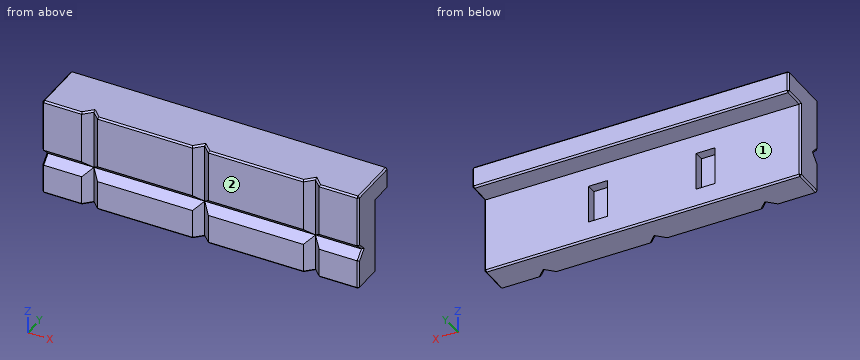
```python
from build123d import *

# Parameters (mm, degrees)
PAD_DEPTH         = 50
POCKET_DEPTH      = 24.001
POCKET_DEPTH_BACK = -7.001
SKETCH002_W       = 6
SKETCH002_H       = 12
POCKET001_DEPTH   = 3
CHAMFER_SIZE      = 0.5


with BuildPart() as part:
    # Sketch → Pad (new body, symmetric)
    with BuildSketch(Plane.YZ):
        Polygon((7, 7), (-10, 7), (-10, -9.5), (-7.5, -12), (-10, -14.5), (-10, -24), (0, -24), (0, 0), (7, 0), align=None)
    extrude(amount=PAD_DEPTH, both=True)

    # Sketch001 → Pocket (cut, two sides)
    with BuildSketch(Plane.XY) as pocket_sk:
        Polygon((-37.5, -10), (-32.5, -10), (-35, -7.5), align=None)
        Polygon((-2.5, -10), (2.5, -10), (0, -7.5), align=None)
        Polygon((32.5, -10), (37.5, -10), (35, -7.5), align=None)
    extrude(amount=-POCKET_DEPTH, mode=Mode.SUBTRACT)
    extrude(pocket_sk.sketch, amount=-POCKET_DEPTH_BACK, mode=Mode.SUBTRACT)

    # Sketch002 → Pocket001 (cut)
    with BuildSketch(Plane.XZ):
        with Locations((-20, -12)):
            Rectangle(SKETCH002_W, SKETCH002_H)
        with Locations((14, -12)):
            Rectangle(SKETCH002_W, SKETCH002_H)
    extrude(amount=POCKET001_DEPTH, mode=Mode.SUBTRACT)

    # Chamfer
    chamfer_edges = [part.edges().sort_by_distance(p)[0] for p in [
        (50, -1.5, 7),
        (50, -10, -1.25),
        (50, -8.75, -10.75),
        (50, -8.75, -13.25),
        (50, -10, -19.25),
        (50, -5, -24),
        (50, 0, -12),
        (50, 3.5, 0),
        (50, 7, 3.5),
        (-50, -1.5, 7),
        (-50, -10, -1.25),
        (-50, -8.75, -10.75),
        (-50, -8.75, -13.25),
        (-50, -10, -19.25),
        (-50, -5, -24),
        (-50, 0, -12),
        (-50, 3.5, 0),
        (-50, 7, 3.5),
        (0, 7, 0),
        (0, 7, 7),
        (-43.75, -10, 7),
        (-36.25, -8.75, 7),
        (-33.75, -8.75, 7),
        (-17.5, -10, 7),
        (-1.25, -8.75, 7),
        (1.25, -8.75, 7),
        (17.5, -10, 7),
        (33.75, -8.75, 7),
        (36.25, -8.75, 7),
        (43.75, -10, 7),
        (0, 0, -24),
        (43.75, -10, -24),
        (36.25, -8.75, -24),
        (33.75, -8.75, -24),
        (17.5, -10, -24),
        (1.25, -8.75, -24),
        (-1.25, -8.75, -24),
        (-17.5, -10, -24),
        (-33.75, -8.75, -24),
        (-36.25, -8.75, -24),
        (-43.75, -10, -24),
    ]]
    chamfer(chamfer_edges, length=CHAMFER_SIZE)


solid = part.part
```
Check sheet for the modelled part. Datum: model origin and axes. Units: mm. Face numbers are marked on the shaded views. A direction names the side the tool comes from. Coordinates: 2 decimals unless noted, no trailing zeros. Order: outer loops, then holes, each group sorted by start corner. A loop starts at its lowest first (then second) coordinate and runs counter-clockwise, first axis right, second up. Notation, with made-up numbers: (73.25, -8.75) -> (94.25, -8.75) arc R12 ccw to (94.25, 4.25) -> close; hole circle Ø6 at (-29.5, 47.25). An arc over 180 degrees is marked (long way). Write item = value, one per line. Start each with the question number.
1) Access from +Z, -Z, +X, -X, +Y, -Y to the whole of each face (thin tool, end or side, straight path). Record for the marked faces 1 and 2.
2) Cross-section at D-D (z = -2). Enter the section's corners in (x, y), then the cut area to 3 significant figures.
3) Cross-section at A-A (z = -17). Enter the section's corners in (x, y), then the cut area to 3 significant figures.
4) Material ranges on L1, parallel to X at y = -0.25, z = -15; L2, parallel to Z at x = -31.5, y = 3; L3, parallel to Y at x = -4, z = -6, recorded low to high.
5) Go/stop test with flat-tipped pins: P1, Ø10, axis at x = -20.5, z = -14, coming from the +Y side; P2, Ø1.8, axis at x = 14.5, z = -13, coming from the +Y side; P3, Ø3.5, axis at x = -17.5, y = 2, coming from the -Z side. Record where each tip stops, or that it passes through.
6) Cross-section at B-B (x = -28). Enter the section's corners in (y, z), then the cut area to 3 significant figures.
7) Cross-section at C-C (y = 3.5). Enter the section's corners in (x, z), then the cut area to 4 significant figures.
Ans:
q1.face_1 = -Z, +X, -X, +Y
q1.face_2 = +Z, -Z, +X, -X, -Y
q2.outline = (-50, -9.5) -> (-49.5, -10) -> (-37.5, -10) -> (-35, -7.5) -> (-32.5, -10) -> (-2.5, -10) -> (0, -7.5) -> (2.5, -10) -> (32.5, -10) -> (35, -7.5) -> (37.5, -10) -> (49.5, -10) -> (50, -9.5) -> (50, -0.5) -> (49.5, 0) -> (-49.5, 0) -> (-50, -0.5) -> close
q2.area = 981 mm²
q3.outline = (-50, -9.5) -> (-49.5, -10) -> (-37.5, -10) -> (-35, -7.5) -> (-32.5, -10) -> (-2.5, -10) -> (0, -7.5) -> (2.5, -10) -> (32.5, -10) -> (35, -7.5) -> (37.5, -10) -> (49.5, -10) -> (50, -9.5) -> (50, -0.5) -> (49.5, 0) -> (17, 0) -> (17, -3) -> (11, -3) -> (11, 0) -> (-17, 0) -> (-17, -3) -> (-23, -3) -> (-23, 0) -> (-49.5, 0) -> (-50, -0.5) -> close
q3.area = 945 mm²
q4.L1 = -49.75 to -23, -17 to 11, 17 to 49.75
q4.L2 = 0 to 7
q4.L3 = -10 to 0
q5.P1 = 0
q5.P2 = -3
q5.P3 = 0
q6.outline = (-10, -23.5) -> (-9.5, -24) -> (-0.5, -24) -> (0, -23.5) -> (0, 0) -> (6.5, 0) -> (7, 0.5) -> (7, 6.5) -> (6.5, 7) -> (-9.5, 7) -> (-10, 6.5) -> (-10, -9.5) -> (-7.5, -12) -> (-10, -14.5) -> close
q6.area = 352 mm²
q7.outline = (-50, 0.5) -> (-49.5, 0) -> (49.5, 0) -> (50, 0.5) -> (50, 6.5) -> (49.5, 7) -> (-49.5, 7) -> (-50, 6.5) -> close
q7.area = 699.5 mm²
